The listing builds one solid part. Answer for the finished solid, in the listing's coordinates (mm). Coordinates: 2 decimals unless noted, no trailing zeros. Order: outer loops, then holes, each group sorted by start corner. A loop starts at its lowest first (then second) coordinate and runs counter-clockwise, first axis right, second up. Notation, with made-up numbers: M -25,76 L 17,76 A34 cw 17,114 Z; hole C 39.5,30.5 d10. An arc over 180 degrees is marked long. One line per item, written item: value. Start each with the question number.
Q1. The part is cut by section A-A on x = -16. Give the vertices of the cut face in (y, z).
Q2. The part is cut by section C-C on z = 2.8. Give the vertices of the cut face in (x, y), then the cut area to 3 significant figures.
Q3. Determine the mould class of faces 1 (the cylindrical face through (0.516, 2.325, 2.348)), 2 (the flat face through (0, -20.206, 2)), 3 (the cylindrical face through (-15.083, -18.447, 2.348)), 4 (the flat face through (13.659, -6.924, 2.348)) for opening direction X: pulls with the +X half, pulls with the -X half, needs draft (parallel to the pull), parting line crosses it, or undercut.
Q4. Each of these flat-tipped pins is pushed along its axis until it touches: pin 1 Ø4.5 at (x, y) = (-16.84, -16.84) entering from +Z; pin 2 Ø2 at (y, z) = (-6, 4) entering from +X. Where does it stop, or does it pass through?
Q5. The part is cut by section D-D on y = 0. Give the vertices of the cut face in (x, z).
Q6. Straight lines are drawn through the part: line 1 along X through (y, z) = (-16.5, 4.4); line 2 along X through (y, z) = (-18.25, 3.8); line 3 along X through (y, z) = (-0.25, 1.35). For each, find the intervals that lie inside material, in ascending order. Write a range as [from, to].
Q7. The part is cut by section B-B on y = -15.5. Give the vertices of the cut face in (x, z), then the cut area to 3 significant figures.
```python
from build123d import *

# Parameters (mm, degrees)
SKETCH1_R           = 2.38125
BOSS_EXTRUDE1_DEPTH = 4.7625


with BuildPart() as part:
    # Sketch1 → Boss-Extrude1 (new body)
    with BuildSketch(Plane.XY):
        Polygon((-26.940768363, -20.205576272), (26.940768363, -20.205576272), (0, 6.735192091), align=None)
        with Locations(Location((0, 0, 0), (0, 0, 180))):
            Circle(SKETCH1_R, mode=Mode.SUBTRACT)
        with Locations(Location((-16.837980227, -16.837980227, 0), (0, 0, 180))):
            Circle(SKETCH1_R, mode=Mode.SUBTRACT)
        with Locations(Location((16.837980227, -16.837980227, 0), (0, 0, 180))):
            Circle(SKETCH1_R, mode=Mode.SUBTRACT)
    extrude(amount=BOSS_EXTRUDE1_DEPTH)


solid = part.part
```
Output:
1. outline: M -20.21,0 L -19.07,0 L -19.07,4.76 L -20.21,4.76 Z; M -14.61,0 L -9.26,0 L -9.26,4.76 L -14.61,4.76 Z
2. outline: M -26.94,-20.21 L 26.94,-20.21 L 0,6.74 Z; hole C -16.84,-16.84 d4.76; hole C 0,0 d4.76; hole C 16.84,-16.84 d4.76
2. area: 672 mm^2
3. face 1: undercut
3. face 2: needs draft
3. face 3: undercut
3. face 4: pulls with the +X half
4. pin 1: passes through
4. pin 2: stops at x = 13.74
5. outline: M -6.74,0 L -2.38,0 L -2.38,4.76 L -6.74,4.76 Z; M 2.38,0 L 6.74,0 L 6.74,4.76 L 2.38,4.76 Z
6. line 1: x = [-23.24, -19.2], [-14.48, 14.48], [19.2, 23.24]
6. line 2: x = [-24.99, -18.76], [-14.92, 14.92], [18.76, 24.99]
6. line 3: x = [-6.99, -2.37], [2.37, 6.99]
7. outline: M -22.24,0 L -18.81,0 L -18.81,4.76 L -22.24,4.76 Z; M -14.87,0 L 14.87,0 L 14.87,4.76 L -14.87,4.76 Z; M 18.81,0 L 22.24,0 L 22.24,4.76 L 18.81,4.76 Z
7. area: 174 mm^2
